from build123d import *

# Parameters (mm, degrees)
SKETCH_R        = 3.25
SKETCH_R_2      = 1.8
PAD_DEPTH       = 5
FILLET_R        = 23
SKETCH001_W     = 30.5
SKETCH001_H     = 8.5
PAD001_DEPTH    = 2
SKETCH002_R     = 1.6
POCKET_DEPTH    = 1.75
POCKET001_DEPTH = 3
POCKET002_DEPTH = 5


with BuildPart() as part:
    # Sketch → Pad (new body)
    with BuildSketch(Plane.XY):
        Polygon((-33.582267, 28.569447), (-3.082267, 28.569447), (-3.082267, 20.069447), (25.8, 20.069447), (25.8, -24), (17.8, -24), (17.8, 14), (-23.069676, 14), (-33.582267, 20.069447), align=None)
        with Locations((-29.332267, 24.319447)):
            Circle(SKETCH_R, mode=Mode.SUBTRACT)
        with Locations((-7.332267, 24.319447)):
            Circle(SKETCH_R, mode=Mode.SUBTRACT)
        with Locations((-21.832267, 18.319447)):
            Circle(SKETCH_R_2, mode=Mode.SUBTRACT)
        with Locations((21.832267, -18.319447)):
            Circle(SKETCH_R_2, mode=Mode.SUBTRACT)
    extrude(amount=PAD_DEPTH)

    # Fillet
    fillet_edges = [part.edges().sort_by_distance(p)[0] for p in [
        (25.8, 20.069447, 2.5),
        (17.8, 14, 2.5),
    ]]
    fillet(fillet_edges, radius=FILLET_R)

    # Sketch001 → Pad001 (new body)
    with BuildSketch(Plane(origin=(0, 0, 0), x_dir=(1, 0, 0), z_dir=(0, 0, -1))):
        with Locations((-18.332267, -24.319447)):
            Rectangle(SKETCH001_W, SKETCH001_H)
    extrude(amount=PAD001_DEPTH)

    # Sketch002 → Pocket (cut)
    with BuildSketch(Plane(origin=(0, 0, -2), x_dir=(1, 0, 0), z_dir=(0, 0, -1))):
        with Locations((-29.332267, -24.319447)):
            Circle(SKETCH002_R)
        with Locations((-7.332267, -24.319447)):
            Circle(SKETCH002_R)
    extrude(amount=-POCKET_DEPTH, mode=Mode.SUBTRACT)

    # Sketch003 → Pocket001 (cut)
    with BuildSketch(Plane(origin=(0, 0, 0), x_dir=(1, 0, 0), z_dir=(0, 0, -1))):
        Polygon((24.733452, 16.644447), (24.733452, 19.994447), (21.832267, 21.669447), (18.931082, 19.994447), (18.931082, 16.644447), (21.832267, 14.969447), align=None)
    extrude(amount=-POCKET001_DEPTH, mode=Mode.SUBTRACT)

    # Sketch004 → Pocket002 (cut)
    with BuildSketch(Plane(origin=(0, 0, -2), x_dir=(1, 0, 0), z_dir=(0, 0, -1))):
        Polygon((-18.931082, -19.994447), (-18.931082, -16.644447), (-21.832267, -14.969447), (-24.733452, -16.644447), (-24.733452, -19.994447), (-21.832267, -21.669447), align=None)
    extrude(amount=-POCKET002_DEPTH, mode=Mode.SUBTRACT)


solid = part.part
Model file for the job. Use its own axes, mm. A direction names the side the tool comes from. Give positions to 0.01 mm unless a question says otherwise; leave off trailing zeros. Loops run counter-clockwise (first coordinate to the right, second up) from the corner with the lowest first, then second, coordinate; pieces in that order, holes last. Notation, with made-up numbers: (15.5, -27.5) -> (60.5, -27.5) arc R15 ccw to (60.5, -8.5) -> close; hole circle Ø9 at (36.25, 14). An arc over 180 degrees is marked (long way). Use a Markdown table: item, result. Add a question column.
(1) Slice it at C-C on y = -13. List the corners of the cut face in (x, z).
(2) Slice it at B-B on x = -13.5. List the corners of the cut face in (y, z).
(3) Tool access for faces 1 (the cylindrical face through (-27.833, 21.436, 2.465)), 2 (the cylindrical face through (18.884, 13.511, 2.535)), 3 (the flat face through (20.36, -15.82, 1.48)), 4 (the flat face through (-14, 14, 2)): list every direction of +Z, -Z, +X, -X, +Y, -Y with a clear straight run to the whole face (end or side of a thin tool).
(4) Slice it at D-D on y = -21. List the corners of the cut face in (x, z), and give its area (3 significant figures).
(5) Wall check: line 1 along Z through (x, y) = (10.5, 15); line 2 along X through (y, z) = (18, 3.5); line 3 along Y through (x, z) = (-13.5, -1.5). Give the ranges that are in metal, low to high.
(6) Drop flat-ended pins along their axis: pin 1 Ø2.5 at (x, y) = (-29.33, 24.32) entering from -Z; pin 2 Ø3.5 at (y, z) = (-19, 1) entering from -X; pin 3 Ø3 at (x, y) = (-7, 23.5) entering from +Z; pin 4 Ø3 at (x, y) = (-21.83, 18.32) entering from -Z. Give the stop position or say it passes through.
(7) Slice it at A-A on z = 2. List the corners of the cut face in (x, y).
(8) Mould opens along Y. For faces 5 (the flat face through (-19, 24, -2)), 6 (the flat face through (-11, 20.069, -1)), 7 (the flat face through (-23.3, 20.82, 0.46)) say: +Y half, -Y half, draft (parallel to the pull), parting line (faces both ways), or undercut.
Filled sheet:
| question | item | result |
|---|---|---|
| 1 | outline | (17.8, 0) -> (25.8, 0) -> (25.8, 5) -> (17.8, 5) -> close |
| 2 | outline | (14, 0) -> (20.07, 0) -> (20.07, -2) -> (28.57, -2) -> (28.57, 5) -> (14, 5) -> close |
| 3 | face 1 | +Z |
| 3 | face 2 | +Z, -Z, +X, +Y |
| 3 | face 3 | -Z |
| 3 | face 4 | +Z, -Z, -X, -Y |
| 4 | outline | (17.8, 0) -> (20.67, 0) -> (20.67, 3) -> (22.99, 3) -> (22.99, 0) -> (25.8, 0) -> (25.8, 5) -> (17.8, 5) -> close |
| 4 | area | 33.0 mm2 |
| 5 | line 1 | 0 to 5 |
| 5 | line 2 | -30 to -23.6, -20.06 to 12.33 |
| 5 | line 3 | 20.07 to 28.57 |
| 6 | pin 1 | z = -0.25 |
| 6 | pin 2 | x = 17.8 |
| 6 | pin 3 | z = 0 |
| 6 | pin 4 | through |
| 7 | outline | (-33.58, 20.07) -> (-23.07, 14) -> (-5.2, 14) arc R23 cw to (17.8, -9) -> (17.8, -24) -> (25.8, -24) -> (25.8, -2.93) arc R23 ccw to (2.8, 20.07) -> (-3.08, 20.07) -> (-3.08, 28.57) -> (-33.58, 28.57) -> close; hole circle Ø6.5 at (-29.33, 24.32); hole (-24.73, 16.64) -> (-21.83, 14.97) -> (-18.93, 16.64) -> (-18.93, 19.99) -> (-21.83, 21.67) -> (-24.73, 19.99) -> close; hole circle Ø6.5 at (-7.33, 24.32); hole (18.93, -19.99) -> (21.83, -21.67) -> (24.73, -19.99) -> (24.73, -16.64) -> (21.83, -14.97) -> (18.93, -16.64) -> close |
| 8 | face 5 | draft |
| 8 | face 6 | -Y half |
| 8 | face 7 | undercut |
